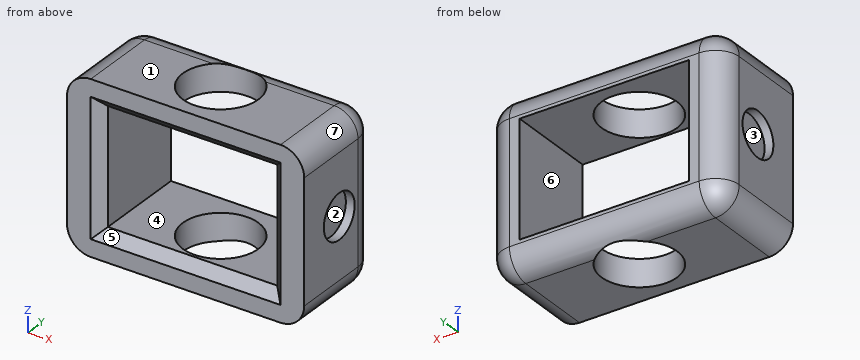
```python
from build123d import *

# Parameters (mm, degrees)
SKETCH1_W               = 70
SKETCH1_H               = 50
BOSS_EXTRUDE1_DEPTH     = 15
SKETCH2_W               = 50
SKETCH2_H               = 34
CUT_EXTRUDE1_DEPTH      = 1
CUT_EXTRUDE1_DEPTH_BACK = 31
FILLET1_R               = 7
CHAMFER1_SIZE           = 3
SKETCH3_R               = 11.15
CUT_EXTRUDE2_DEPTH      = 1
CUT_EXTRUDE2_DEPTH_BACK = 51
SKETCH4_R               = 6.6
CUT_EXTRUDE3_DEPTH      = 2.6


with BuildPart() as part:
    # Sketch1 → Boss-Extrude1 (new body, symmetric)
    with BuildSketch(Plane(origin=(0, 0, 0), x_dir=(1, 0, 0), z_dir=(0, 1, 0))):
        Rectangle(SKETCH1_W, SKETCH1_H)
    extrude(amount=BOSS_EXTRUDE1_DEPTH, both=True)

    # Sketch2 → Cut-Extrude1 (cut, two sides)
    with BuildSketch(Plane.XZ.offset(15)) as cut_extrude1_sk:
        Rectangle(SKETCH2_W, SKETCH2_H)
    extrude(amount=CUT_EXTRUDE1_DEPTH, mode=Mode.SUBTRACT)
    extrude(cut_extrude1_sk.sketch, amount=-CUT_EXTRUDE1_DEPTH_BACK, mode=Mode.SUBTRACT)

    # Fillet1
    fillet1_edges = [part.edges().sort_by_distance(p)[0] for p in [
        (-35, 15, 0),
        (0, 15, 25),
        (35, 15, 0),
        (0, 15, -25),
        (35, 0, 25),
        (-35, 0, 25),
        (-35, 0, -25),
        (35, 0, -25),
    ]]
    fillet(fillet1_edges, radius=FILLET1_R)

    # Chamfer1
    chamfer1_edges = [part.edges().sort_by_distance(p)[0] for p in [
        (0, -15, 17),
        (-25, -15, 0),
        (0, -15, -17),
        (25, -15, 0),
    ]]
    chamfer(chamfer1_edges, length=CHAMFER1_SIZE)

    # Sketch3 → Cut-Extrude2 (cut, two sides)
    with BuildSketch(Plane(origin=(0, 0, -25), x_dir=(-1, 0, 0), z_dir=(0, 0, -1))) as cut_extrude2_sk:
        Circle(SKETCH3_R)
    extrude(amount=CUT_EXTRUDE2_DEPTH, mode=Mode.SUBTRACT)
    extrude(cut_extrude2_sk.sketch, amount=-CUT_EXTRUDE2_DEPTH_BACK, mode=Mode.SUBTRACT)

    # Sketch4 → Cut-Extrude3 (cut)
    with BuildSketch(Plane(origin=(35, 0, 0), x_dir=(0, 0, -1), z_dir=(1, 0, 0))):
        Circle(SKETCH4_R)
    cut_extrude3 = extrude(amount=-CUT_EXTRUDE3_DEPTH, mode=Mode.SUBTRACT)

    # Mirror1: Cut-Extrude3 across plane
    add(cut_extrude3.mirror(Plane(origin=(0, 0, 0), x_dir=(0, 0, 1), z_dir=(1, 0, 0))), mode=Mode.SUBTRACT)


solid = part.part
```
The model under review builds one solid part; all positions refer to its coordinate system, in mm. Face numbers are marked on the shaded views. A direction names the side the tool comes from. Give positions to 0.01 mm unless a question says otherwise; leave off trailing zeros. Write each loop counter-clockwise with the first axis right and the second up, starting at its lowest first coordinate (ties: lowest second). Pieces come first, ordered by that corner, then holes. Notation, with made-up numbers: M -40,-1.5 L -9,-1.5 A13 ccw -9,20.5 Z; hole C -19,-39.5 d7. An arc over 180 degrees is marked long. Write item = value, one per line. Start each with the question number.
Q1. Clearance check with flat-ended pins moving along their axes: pin 1 (5 mm diameter, centred on x = 11, y = 0, fed in from +Z); pin 2 (12 mm diameter, centred on y = 0, z = 0, fed in from +X); pin 3 (8 mm diameter, centred on x = 22.5, z = -4, fed in from -Y); pin 4 (12 mm diameter, centred on x = -21, z = -6, fed in from -Y). State where each tip first meets the part, or that it passes through.
Q2. We need section C-C (z = 0). State the section outline as (x, y) points, plus the area to 3 significant figures.
Q3. Machinability: for the marked faces 5, 6 and 7, which of the approach directions +Z, -Z, +X, -X, +Y, -Y give a long, thin tool a straight path to every point of the face, cutting with its end or side? Answer none if there is none.
Q4. We need section A-A (x = 20). State the section outline as (y, z) points.
Q5. For line 1 (Z direction, x = -11.5, y = 4); line 2 (X direction, y = 3.5, z = 10.5); line 3 (X direction, y = 0, z = 6), list the stretches that pass through material, from the lowest coordinate up.
Q6. We need section B-B (y = 0). State the section outline as (x, z) points.
Q7. Mouldability with a two-part tool opening along X and no side actions: class the marked faces 1, 2, 3 and 4 as released by +X, released by -X, zero draft, split by the parting line, or undercut.
Q8. We need section D-D (x = 4). State the section outline as (y, z) points.
Result set:
q1.pin_1 = 25
q1.pin_2 = 32.4
q1.pin_3 = -13.5
q1.pin_4 = -14
q2.outline = M -35,-15 L -28,-15 L -25,-12 L -25,15 L -28,15 A7 ccw -35,8 L -35,6.6 L -32.4,6.6 L -32.4,-6.6 L -35,-6.6 Z; M 25,-12 L 28,-15 L 35,-15 L 35,-6.6 L 32.4,-6.6 L 32.4,6.6 L 35,6.6 L 35,8 A7 ccw 28,15 L 25,15 Z
q2.area = 501 mm2
q3.face_5 = -Y
q3.face_6 = +Y, -Y
q3.face_7 = +Z, +X, +Y, -Y
q4.outline = M -15,-25 L 8,-25 A7 ccw 15,-18 L 15,-17 L -12,-17 L -15,-20 Z; M -15,20 L -12,17 L 15,17 L 15,18 A7 ccw 8,25 L -15,25 Z
q5.line_1 = -25 to -17, 17 to 25
q5.line_2 = -35 to -25, 25 to 35
q5.line_3 = -32.4 to -25, 25 to 32.4
q6.outline = M -35,-18 A7 ccw -28,-25 L -11.15,-25 L -11.15,-17 L -25,-17 L -25,17 L -11.15,17 L -11.15,25 L -28,25 A7 ccw -35,18 L -35,6.6 L -32.4,6.6 L -32.4,-6.6 L -35,-6.6 Z; M 11.15,-25 L 28,-25 A7 ccw 35,-18 L 35,-6.6 L 32.4,-6.6 L 32.4,6.6 L 35,6.6 L 35,18 A7 ccw 28,25 L 11.15,25 L 11.15,17 L 25,17 L 25,-17 L 11.15,-17 Z
q7.face_1 = zero draft
q7.face_2 = released by +X
q7.face_3 = released by -X
q7.face_4 = undercut
q8.outline = M -15,-25 L -10.41,-25 L -10.41,-17 L -12,-17 L -15,-20 Z; M -15,20 L -12,17 L -10.41,17 L -10.41,25 L -15,25 Z; M 10.41,-24.57 A7 ccw 15,-18 L 15,-17 L 10.41,-17 Z; M 10.41,17 L 15,17 L 15,18 A7 ccw 10.41,24.57 Z
